CAD build for the part. Positions are in the model's coordinates, mm. Coordinates: 2 decimals unless noted, no trailing zeros. Write each loop counter-clockwise with the first axis right and the second up, starting at its lowest first coordinate (ties: lowest second). Pieces come first, ordered by that corner, then holes. Notation, with made-up numbers: (76.25, 9) - (133.25, 9) arc R37 cw to (133.25, 48) - close; hole circle Ø10 at (36, 32.25). An arc over 180 degrees is marked (long way). Answer in a Markdown table with one row per item. Add a question column.
Q1. Band-saw the part on A-A (x = -31). List the corners of the cut face in (y, z), and give its area (3 significant figures).
Q2. Band-saw the part on B-B (z = 1.7). List the corners of the cut face in (x, y), and give its area (3 significant figures).
Q3. Drill centre lines: line 1 along Y through (x, z) = (-31, 2.1); line 2 along X through (y, z) = (-4, 1.1); line 3 along X through (y, z) = (-3.75, 2). Where is each one in solid material? Low to high. Write a range as from..to.
Q4. Pin check, flat tip, straight feed: pin 1 (7 mm diameter, centred on x = -31, y = -2.5, fed in from +Z). Stop position of the tip, or through.
```python
from build123d import *

# Parameters (mm, degrees)
SKETCH1_W           = 134
SKETCH1_H           = 15
BOSS_EXTRUDE1_DEPTH = 3
SKETCH4_R           = 3
CUT_EXTRUDE1_DEPTH  = 3
SKETCH2_R           = 3
CUT_EXTRUDE2_DEPTH  = 3


with BuildPart() as part:
    # Sketch1 → Boss-Extrude1 (new body)
    with BuildSketch(Plane.XY):
        Rectangle(SKETCH1_W, SKETCH1_H)
    extrude(amount=BOSS_EXTRUDE1_DEPTH)

    # Sketch4 → Cut-Extrude1 (cut)
    with BuildSketch(Plane(origin=(0, 0, 0), x_dir=(-1, 0, 0), z_dir=(0, 0, -1))):
        with Locations((-31, -2.5)):
            Circle(SKETCH4_R)
    extrude(amount=-CUT_EXTRUDE1_DEPTH, mode=Mode.SUBTRACT)

    # Sketch2 → Cut-Extrude2 (cut)
    with BuildSketch(Plane(origin=(0, 0, 0), x_dir=(-1, 0, 0), z_dir=(0, 0, -1))):
        with Locations((31, -2.5)):
            Circle(SKETCH2_R)
    extrude(amount=-CUT_EXTRUDE2_DEPTH, mode=Mode.SUBTRACT)


solid = part.part
```
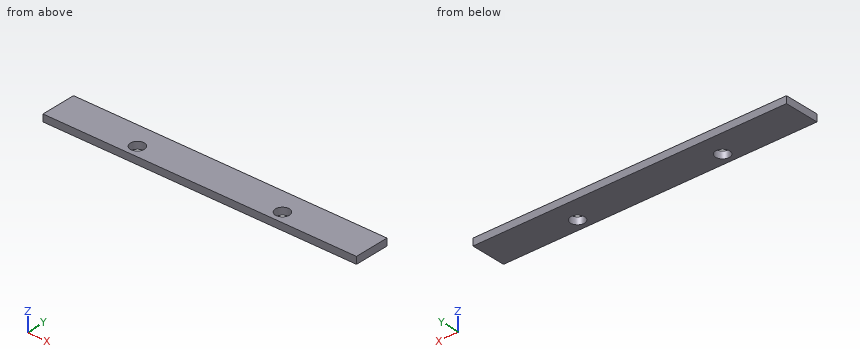
Checked values:
| question | item | result |
|---|---|---|
| 1 | outline | (-7.5, 0) - (-5.5, 0) - (-5.5, 3) - (-7.5, 3) - close; (0.5, 0) - (7.5, 0) - (7.5, 3) - (0.5, 3) - close |
| 1 | area | 27.0 mm² |
| 2 | outline | (-67, -7.5) - (67, -7.5) - (67, 7.5) - (-67, 7.5) - close; hole circle Ø6 at (-31, -2.5); hole circle Ø6 at (31, -2.5) |
| 2 | area | 1,950 mm² |
| 3 | line 1 | y = -7.5..-5.5, 0.5..7.5 |
| 3 | line 2 | x = -67..-33.6, -28.4..28.4, 33.6..67 |
| 3 | line 3 | x = -67..-33.73, -28.27..28.27, 33.73..67 |
| 4 | pin 1 | stops at z = 3 |
